Source: CAD feature listing. Evaluate the final solid. Frame: model axes, mm. Face numbers are marked on the shaded views. A direction names the side the tool comes from. Round coordinates to 2 decimals unless told otherwise and drop trailing zeros. Write each loop counter-clockwise with the first axis right and the second up, starting at its lowest first coordinate (ties: lowest second). Pieces come first, ordered by that corner, then holes. Notation, with made-up numbers: (-30.5, 19) -> (11.5, 19) arc R32 cw to (11.5, 58) -> close; hole circle Ø8 at (-30.75, 61). An arc over 180 degrees is marked (long way). Put each result on its own line as item: value.
```python
from build123d import *

# Parameters (mm, degrees)
BOSS_EXTRUDE1_DEPTH = 5
BOSS_EXTRUDE2_DEPTH = 6
FILLET1_R           = 1.5


with BuildPart() as part:
    # Sketch1 → Boss-Extrude1 (new body)
    with BuildSketch(Plane.XY):
        with BuildLine():
            Line((0, 0), (0, 11.493077271))
            ThreePointArc((0, 11.493077271), (-0.413175911, 11.985481147), (-0.96984631, 11.664087342))
            Line((-0.96984631, 11.664087342), (-4.900710246, 0.864127441))
            Line((-4.900710246, 0.864127441), (-5.840402867, 1.206147584))
            Line((-5.840402867, 1.206147584), (-0.939692621, 14.670738324))
            ThreePointArc((-0.939692621, 14.670738324), (0.173648178, 15.313525933), (1, 14.32871818))
            Line((1, 14.32871818), (1, 0))
            Line((1, 0), (0, 0))
        make_face()
    extrude(amount=BOSS_EXTRUDE1_DEPTH)

    # Sketch2 → Boss-Extrude2 (add)
    with BuildSketch(Plane(origin=(1, 0, 0), x_dir=(0, 0, -1), z_dir=(1, 0, 0))):
        with BuildLine():
            ThreePointArc((-2.5, 5.5), (-4.267766953, 1.232233047), (0, 3))
            ThreePointArc((0, 3), (-0.732233047, 4.767766953), (-2.5, 5.5))
        make_face()
    extrude(amount=BOSS_EXTRUDE2_DEPTH)

    # Fillet1
    fillet1_edges = [part.edges().sort_by_distance(p)[0] for p in [
        (7, 3, 5),
    ]]
    fillet(fillet1_edges, radius=FILLET1_R)


solid = part.part
```
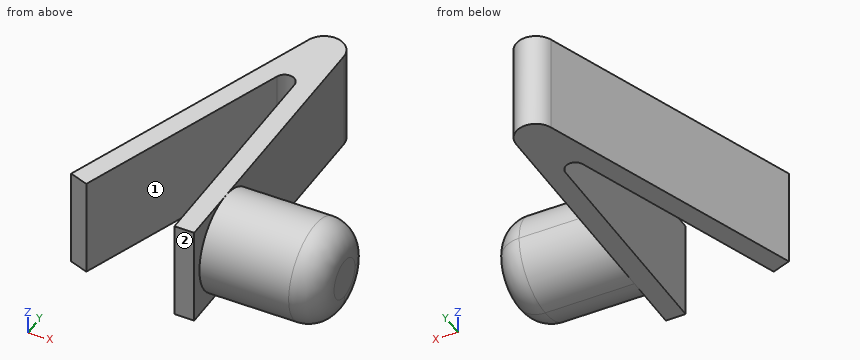
Q1. Cut plane A-A on y = 11. Output: boundary loops of the cut face in (x, z), and give its area (3 significant figures).
Ans:
outline: (-2.28, 0) -> (-1.21, 0) -> (-1.21, 5) -> (-2.28, 5) -> close; (0, 0) -> (1, 0) -> (1, 5) -> (0, 5) -> close
area: 10.3 mm^2
Q2. Material intervals for line 1 (Y direction, x = 3.25, z = 2.5); line 2 (X direction, y = 11.25, z = 2.35); line 3 (X direction, y = 2.5, z = 3.7), sorted ascending. Write a range as [from, to].
Ans:
line 1: y = [0.5, 5.5]
line 2: x = [-2.18, -1.12], [0, 1]
line 3: x = [-5.37, -4.31], [0, 6.97]
Q3. Cut plane B-B on x = -2.75. Output: boundary loops of the cut face in (y, z).
Ans:
outline: (6.77, 0) -> (9.7, 0) -> (9.7, 5) -> (6.77, 5) -> close
Q4. Pin query (flat end, axial travel): pin 1 (1 mm diameter, centred on x = 2.5, z = 2, fed in from +Y); pin 2 (1.5 mm diameter, centred on y = 7, z = 2.5, fed in from +X); pin 3 (1.5 mm diameter, centred on y = 7.5, z = 1.5, fed in from -X). Return the tip coordinate at first contact, or that it passes through.
Ans:
pin 1: stops at y = 5.5
pin 2: stops at x = 1
pin 3: stops at x = -3.82
Q5. Reachability of the marked faces 1 and 2 from +Z, -Z, +X, -X, +Y, -Y: full face, straight path, thin tool, end or side. Return the list, or none.
Ans:
face 1: +Z, -Z, -Y
face 2: +Z, -Z, +X, -X, -Y
